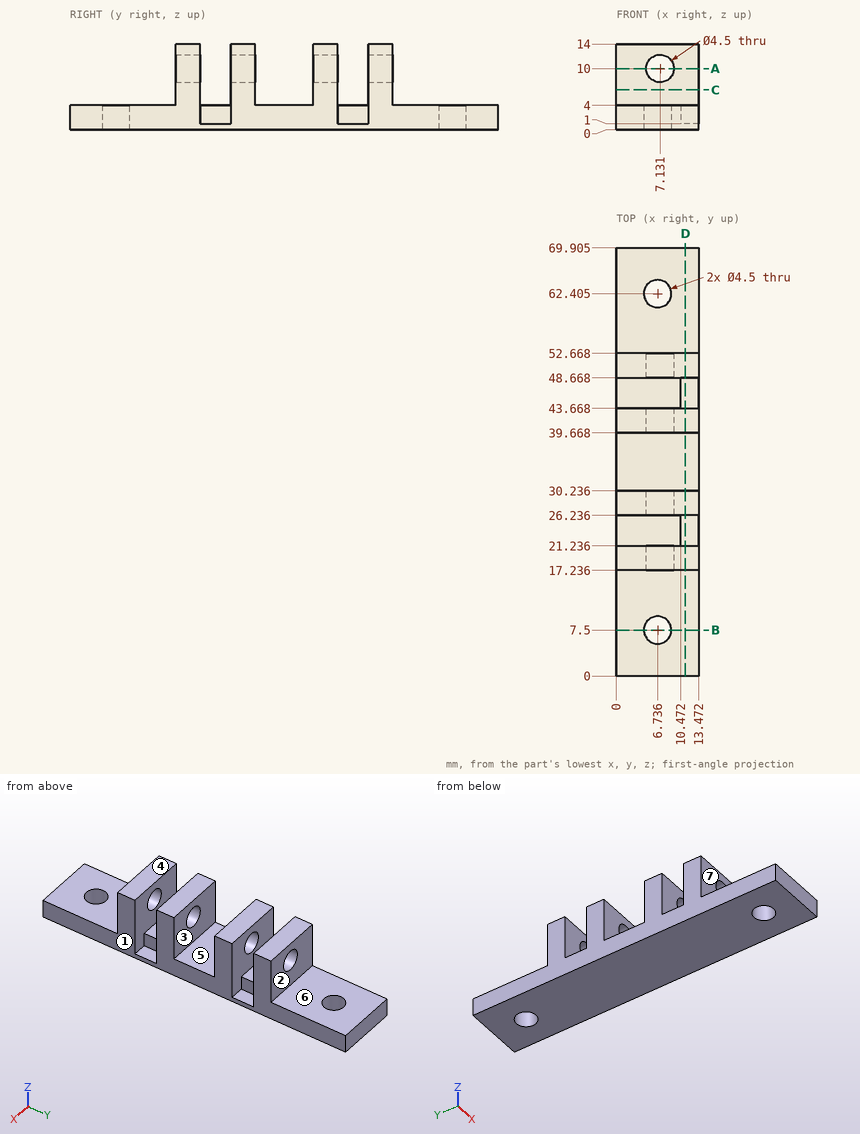
Answer from the drawing. Dimensions are ordinates in mm from the lowest x, y and z of the part. A direction names the side the tool comes from. Round coordinates to 2 decimals unless told otherwise and drop trailing zeros. Loops run counter-clockwise (first coordinate to the right, second up) from the corner with the lowest first, then second, coordinate; pieces in that order, holes last. Notation, with made-up numbers: M 80.5,3.25 L 102.5,3.25 A14 cw 102.5,27.25 Z; hole C -24,62.5 d3. An arc over 180 degrees is marked long. One line per question, with ' | ' between items. Start each with the question number.
(1) A cutting plane is placed at D-D on x = 11.25. Write down the section's boundary in (y, z) (1 decimal).
(2) A cutting plane is placed at B-B on y = 7.5. Write down the section's boundary in (x, z) (1 decimal), plus the area to 3 significant figures.
(3) A cutting plane is placed at C-C on z = 6.5. Write down the section's boundary in (x, y).
(4) A cutting plane is placed at A-A on z = 10. Give the number of separate pieces and of enclosed holes in the cut face.
(5) For a pull along Y with two mould halves and no side action, classify the marked faces 1, 2 and 3 as released by +Y, released by -Y, zero draft, split by the parting line, or undercut.
(6) Flat-ended cylindrical pins translate along their axes: pin 1 Ø7 at (x, y) = (6.74, 62.4) entering from +Z; pin 2 Ø2 at (x, z) = (4, 7) entering from -Y; pin 3 Ø5 at (x, z) = (6.5, 10) entering from +Y; pin 4 Ø8 at (y, z) = (30, 9.5) entering from -X. Find the tip coordinate at first contact, or state that the pin passes through.
(7) Find the intervals of material crossed by line 1 (Y direction, x = 6.5, z = 3) (1 decimal); line 2 (Y direction, x = 12.25, z = 6.5); line 3 (X direction, y = 7.5, z = 2.1) (1 decimal), in increasing order.
(8) A tool of negligible diameter and unlimited length cuts with its end or side. For the marked faces 4, 5, 6 and 7, from which of +Z, -Z, +X, -X, +Y, -Y can it reach the whole face along a straight path? Write none if from no direction.
Geometry check:
1) outline: M 0,0 L 69.9,0 L 69.9,4 L 52.7,4 L 52.7,14 L 48.7,14 L 48.7,1 L 43.7,1 L 43.7,14 L 39.7,14 L 39.7,4 L 30.2,4 L 30.2,14 L 26.2,14 L 26.2,1 L 21.2,1 L 21.2,14 L 17.2,14 L 17.2,4 L 0,4 Z
2) outline: M 0,0 L 4.5,0 L 4.5,4 L 0,4 Z; M 9,0 L 13.5,0 L 13.5,4 L 9,4 Z | area: 35.9 mm²
3) outline: M 0,17.24 L 13.47,17.24 L 13.47,21.24 L 0,21.24 Z; M 0,26.24 L 13.47,26.24 L 13.47,30.24 L 0,30.24 Z; M 0,39.67 L 13.47,39.67 L 13.47,43.67 L 0,43.67 Z; M 0,48.67 L 13.47,48.67 L 13.47,52.67 L 0,52.67 Z
4) separate pieces: 8 | enclosed holes: 0
5) face 1: zero draft | face 2: released by +Y | face 3: undercut
6) pin 1: stops at z = 4 | pin 2: stops at y = 17.24 | pin 3: stops at y = 52.67 | pin 4: stops at x = 0
7) line 1: y = 0 to 5.3, 9.7 to 60.2, 64.6 to 69.9 | line 2: y = 17.24 to 21.24, 26.24 to 30.24, 39.67 to 43.67, 48.67 to 52.67 | line 3: x = 0 to 4.5, 9 to 13.5
8) face 4: +Z, +X, -X, +Y, -Y | face 5: +Z, +X, -X | face 6: +Z, +X, -X, +Y | face 7: +Z, +X, -X, -Y
